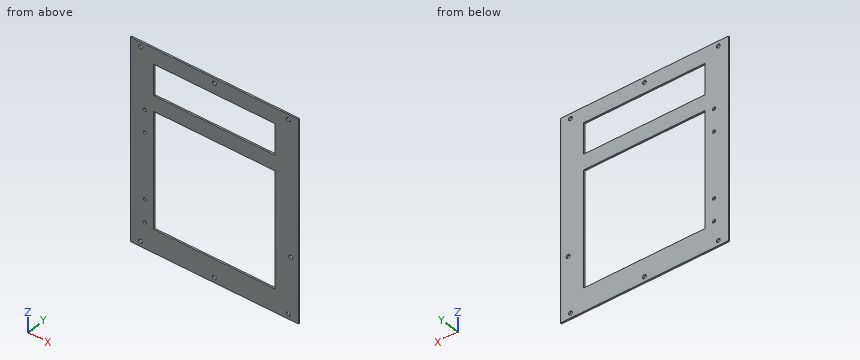
from build123d import *

# Parameters (mm, degrees)
SKETCH_1_W          = 216
SKETCH_1_H          = 260
EXTRUDE_1_DEPTH     = 2
SKETCH_3_W          = 156
SKETCH_3_H          = 150
SKETCH_3_H_2        = 40
CUT_EXTRUDE_2_DEPTH = 2
SKETCH_5_R          = 2.5
CUT_EXTRUDE_3_DEPTH = 2
MM_2_D              = 4
MM_2_DEPTH          = 10
MM_2_TIP            = 1.201721238
MM_4_D              = 5
MM_4_DEPTH          = 380


with BuildPart() as part:
    # 草图1 → 凸台-拉伸1 (new body)
    with BuildSketch(Plane(origin=(0, 0, 0), x_dir=(1, 0, 0), z_dir=(0, 1, 0))):
        Rectangle(SKETCH_1_W, SKETCH_1_H)
    extrude(amount=EXTRUDE_1_DEPTH)

    # 草图3 → 切除-拉伸2 (cut)
    with BuildSketch(Plane.XZ):
        with Locations((0, -25)):
            Rectangle(SKETCH_3_W, SKETCH_3_H)
        with Locations((0, 90)):
            Rectangle(SKETCH_3_W, SKETCH_3_H_2)
    extrude(amount=-CUT_EXTRUDE_2_DEPTH, mode=Mode.SUBTRACT)

    # 草图5 → 切除-拉伸3 (cut)
    with BuildSketch(Plane.XZ):
        with Locations(Location((98, -50, 0), (0, 0, 270))):
            Circle(SKETCH_5_R)
    extrude(amount=-CUT_EXTRUDE_3_DEPTH, mode=Mode.SUBTRACT)

    # 大小mm 暗销孔2
    with Locations(Plane(origin=(45.636831669, 3.8, 442.05931397), x_dir=(0.07852837759024343, 0, 0.9969118787099711), z_dir=(0, 1, 0))):
        with Locations((-404.949854974, -103.656881575), (-403.897574678, -90.298262111), (-432.80801916, -88.020939161), (-433.860299457, -101.379558625), (-547.50825363, -92.42732358), (-518.597809147, -94.70464653), (-517.545528888, -81.346027355), (-546.45597337, -79.068704405)):
            Hole(MM_2_D / 2, depth=MM_2_DEPTH)
            with Locations((0, 0, -(MM_2_DEPTH + MM_2_TIP / 2))):  # 118° drill point
                Cone(0, MM_2_D / 2, MM_2_TIP, mode=Mode.SUBTRACT)

    # 大小mm 暗销孔4
    with Locations(Plane(origin=(45.636831669, -378, 442.05931397), x_dir=(-0.07852837759024327, 0, -0.9969118787099712), z_dir=(0, -1, 0))):
        with Locations((559.93638869, 93.623184237), (567.396584561, -1.08344424), (574.856780432, -95.790072718), (313.699154648, 74.226674972), (321.159350519, -20.479953505), (328.61954639, -115.186581983)):
            Hole(MM_4_D / 2, depth=MM_4_DEPTH)


solid = part.part
CAD build for the part. Positions are in the model's coordinates, mm. Round coordinates to 2 decimals unless told otherwise and drop trailing zeros. Order: outer loops, then holes, each group sorted by start corner. A loop starts at its lowest first (then second) coordinate and runs counter-clockwise, first axis right, second up. Notation, with made-up numbers: M -8.75,70 L 30.25,70 A25 cw 30.25,93 Z; hole C 10,-29 d6. An arc over 180 degrees is marked long. Use one line per item in the form item = value.
Q1. Saw through at A-A on z = 27.5. Give the cut face in (x, y), then the cut area to 3 significant figures.
Recorded:
outline = M -108,0 L -78,0 L -78,2 L -108,2 Z; M 78,0 L 108,0 L 108,2 L 78,2 Z
area = 120 mm^2
Q2. Probe L1, parallel to Z at x = 95, y = 0.95; L2, parallel to X at y = 0.8, z = 123.5; L3, parallel to Z at x = -22, y = 0.95. List the from-to ranges inside material, lowest first.
Recorded:
L1 = -130 to -126, -121 to 121, 126 to 130
L2 = -108 to -97.5, -92.5 to -2.5, 2.5 to 92.5, 97.5 to 108
L3 = -130 to -100, 50 to 70, 110 to 130
Q3. Saw through at B-B on x = 11.5. Give the cut face in (y, z).
Recorded:
outline = M 0,-130 L 2,-130 L 2,-100 L 0,-100 Z; M 0,50 L 2,50 L 2,70 L 0,70 Z; M 0,110 L 2,110 L 2,130 L 0,130 Z
Q4. Saw through at C-C on y = 0.3. State how many separate pieces and enclosed holes the cut face has, then the cut area to 3 significant figures.
Recorded:
separate_pieces = 1
enclosed_holes = 13
area = 26,300 mm^2
